from build123d import *

# Parameters (mm, degrees)
EXTRUDE_1_DEPTH = 12
FILLET_2_R      = 10
SKETCH_2_R      = 5


with BuildPart() as part:
    # 草图1 → 凸台-拉伸1 (new body)
    with BuildSketch(Plane(origin=(0, 0, 0), x_dir=(1, 0, 0), z_dir=(0, 1, 0))):
        Polygon((0, 0), (0, -40), (50, -40), (50, -20), (20, -20), (20, 0), align=None)
    extrude(amount=EXTRUDE_1_DEPTH)

    # 圆角2
    fillet_2_edges = [part.edges().sort_by_distance(p)[0] for p in [
        (20, 6, 20),
        (0, 6, 40),
    ]]
    fillet(fillet_2_edges, radius=FILLET_2_R)

    # 切除-扫描1: sweep along a path in 草图4
    with BuildLine(Plane(origin=(0, 6, 0), x_dir=(-1, 0, 0), z_dir=(0, -1, 0))) as sweep_1_path:
        Line((-10, 3.270515342), (-10, -20))
        ThreePointArc((-10, -20), (-12.928932188, -27.071067812), (-20, -30))
        Line((-20, -30), (-53.042337367, -30))
    # 草图2 → 切除-扫描1 (sweep, cut)
    with BuildSketch(Plane(origin=(0, 0, 0), x_dir=(-1, 0, 0), z_dir=(0, 0, -1))):
        with Locations((-10, 6)):
            Circle(SKETCH_2_R)
    sweep(path=sweep_1_path.line, mode=Mode.SUBTRACT)


solid = part.part
Part model, mm, in its own coordinate system. A direction names the side the tool comes from. Give positions to 0.01 mm unless a question says otherwise; leave off trailing zeros. Order: outer loops, then holes, each group sorted by start corner. A loop starts at its lowest first (then second) coordinate and runs counter-clockwise, first axis right, second up. Notation, with made-up numbers: (86.5, 86.25) -> (145.5, 86.25) arc R25 cw to (145.5, 109.25) -> close; hole circle Ø3 at (21, -37). An arc over 180 degrees is marked (long way). Use one line per item in the form item = value.
(1) Tool access for faces 1 (the face through (15, 3, 0)), 2 (the face through (5.381, 7.915, 10.14)), 3 (the face through (40, 6, 20)): list every direction of +Z, -Z, +X, -X, +Y, -Y with a clear straight run to the whole face (end or side of a thin tool).
Solution:
face_1 = -Z, +X, -X, +Y, -Y
face_2 = -Z
face_3 = -Z, +X, +Y, -Y
(2) Pull direction Z, two halves, no side cores. Call faces 4 (the face through (35, 6, 25)), 5 (the face through (23.01, 6.08, 17.15)), 6 (the face through (0, 6, 15)): +Z half, -Z half, draft (parallel to the pull), parting line (faces both ways), or undercut.
Solution:
face_4 = undercut
face_5 = -Z half
face_6 = draft
(3) Saw through at A-A (y = 6). Write the cut outline in (x, z).
Solution:
outline = (0, 0) -> (5, 0) -> (5, 20) arc R15 cw to (20, 35) -> (50, 35) -> (50, 40) -> (10, 40) arc R10 ccw to (0, 30) -> close; (15, 0) -> (20, 0) -> (20, 10) arc R10 cw to (30, 20) -> (50, 20) -> (50, 25) -> (20, 25) arc R5 ccw to (15, 20) -> close
(4) Saw through at D-D (y = 8.5). Write the cut outline in (x, z), then the cut area to 3 significant figures.
Solution:
outline = (0, 0) -> (5.67, 0) -> (5.67, 20) arc R14.33 cw to (20, 34.33) -> (50, 34.33) -> (50, 40) -> (10, 40) arc R10 ccw to (0, 30) -> close; (14.33, 0) -> (20, 0) -> (20, 10) arc R10 cw to (30, 20) -> (50, 20) -> (50, 25.67) -> (20, 25.67) arc R5.67 ccw to (14.33, 20) -> close
area = 831 mm²
(5) Drill centre lines: line 1 (Y direction, x = 10, z = 11.25); line 2 (X direction, y = 6, z = 4.5); line 3 (X direction, y = 9, z = 8). Where is each one in solid material? Low to high. Write a range as from..to.
Solution:
line_1 = 0..1, 11..12
line_2 = 0..5, 15..20
line_3 = 0..6, 14..20
(6) Saw through at B-B (x = 33). Write the cut outline in (y, z).
Solution:
outline = (0, 20) -> (12, 20) -> (12, 40) -> (0, 40) -> close; hole circle Ø10 at (6, 30)
(7) Flat gauge pins, fed straight in: P1, Ø1.5, axis at x = 6, y = 4.5, coming from the +Z side; P2, Ø2, axis at x = 24.5, y = 6, coming from the -Z side; P3, Ø6, axis at x = 40.5, y = 4, coming from the -Z side. Where does each tip first touch, or does it go through?
Solution:
P1 = 39.46
P2 = 17.6
P3 = 20
(8) Saw through at C-C (z = 4). Write the cut outline in (x, y), then the cut area to 3 significant figures.
Solution:
outline = (0, 0) -> (20, 0) -> (20, 12) -> (0, 12) -> close; hole circle Ø10 at (10, 6)
area = 161 mm²
